```python
from build123d import *

# Parameters (mm, degrees)
F0_R     = 4.35
F0_R_2   = 5
F1_DEPTH = 4.3


with BuildPart() as f1:
    # F0 (on Right) → F1 (new body)
    with BuildSketch(Plane.YZ):
        with BuildLine():
            Line((-22.1, 0), (-5, 0))
            ThreePointArc((-5, 0), (-1.464466, 1.464466), (0, 5))
            Line((0, 5), (0, 29.037729))
            ThreePointArc((0, 29.037729), (-0.662326, 31.524611), (-2.473833, 33.352642))
            Line((-2.473833, 33.352642), (-32.57476, 50.975239))
            ThreePointArc((-32.57476, 50.975239), (-33.70512, 51.245677), (-34.79499, 50.841905))
            Line((-34.79499, 50.841905), (-42.052337, 45.329218))
            Line((-42.052337, 45.329218), (-98.45379, 75.262621))
            ThreePointArc((-98.45379, 75.262621), (-98.549794, 75.301433), (-98.651734, 75.319636))
            Line((-98.651734, 75.319636), (-104.857779, 75.773284))
            ThreePointArc((-104.857779, 75.773284), (-104.881835, 75.769417), (-104.901607, 75.755178))
            ThreePointArc((-104.901607, 75.755178), (-104.997551, 75.587599), (-105.022838, 75.396161))
            Line((-105.022838, 75.396161), (-104.855972, 72.750564))
            ThreePointArc((-104.855972, 72.750564), (-104.882304, 72.556066), (-104.98147, 72.386689))
            ThreePointArc((-104.98147, 72.386689), (-105.0797, 72.27604), (-105.177659, 72.165152))
            ThreePointArc((-105.177659, 72.165152), (-105.519248, 71.996856), (-105.880288, 72.117919))
            Line((-105.880288, 72.117919), (-107.19123, 73.254305))
            ThreePointArc((-107.19123, 73.254305), (-107.768907, 72.57831), (-108.336982, 71.894228))
            ThreePointArc((-108.336982, 71.894228), (-108.432061, 71.710527), (-108.44465, 71.504063))
            Line((-108.44465, 71.504063), (-108.056233, 68.888956))
            ThreePointArc((-108.056233, 68.888956), (-108.06619, 68.692429), (-108.151209, 68.514964))
            ThreePointArc((-108.151209, 68.514964), (-108.239818, 68.396849), (-108.328139, 68.27852))
            ThreePointArc((-108.328139, 68.27852), (-108.65472, 68.082686), (-109.024498, 68.17363))
            Line((-109.024498, 68.17363), (-110.424503, 69.198289))
            ThreePointArc((-110.424503, 69.198289), (-110.941832, 68.480942), (-111.449037, 67.756402))
            ThreePointArc((-111.449037, 67.756402), (-111.530067, 67.558002), (-111.520592, 67.343902))
            Line((-111.520592, 67.343902), (-110.867678, 64.891617))
            ThreePointArc((-110.867678, 64.891617), (-110.856617, 64.687221), (-110.92839, 64.495521))
            ThreePointArc((-110.92839, 64.495521), (-111.004676, 64.374709), (-111.080678, 64.253718))
            ThreePointArc((-111.080678, 64.253718), (-111.390502, 64.032323), (-111.766382, 64.093319))
            Line((-111.766382, 64.093319), (-113.244054, 65.002399))
            ThreePointArc((-113.244054, 65.002399), (-113.70347, 64.243719), (-114.152157, 63.478645))
            ThreePointArc((-114.152157, 63.478645), (-114.216631, 63.278226), (-114.192891, 63.069034))
            Line((-114.192891, 63.069034), (-113.365453, 60.614331))
            ThreePointArc((-113.365453, 60.614331), (-113.340818, 60.415154), (-113.396489, 60.222336))
            ThreePointArc((-113.396489, 60.222336), (-113.463838, 60.093583), (-113.53088, 59.964669))
            ThreePointArc((-113.53088, 59.964669), (-113.821693, 59.718835), (-114.201286, 59.749091))
            Line((-114.201286, 59.749091), (-115.74793, 60.535116))
            ThreePointArc((-115.74793, 60.535116), (-116.14419, 59.74162), (-116.529237, 58.942622))
            ThreePointArc((-116.529237, 58.942622), (-116.577215, 58.737628), (-116.536559, 58.531056))
            Line((-116.536559, 58.531056), (-115.512428, 56.151691))
            ThreePointArc((-115.512428, 56.151691), (-115.471694, 55.955174), (-115.511515, 55.758471))
            ThreePointArc((-115.511515, 55.758471), (-115.568182, 55.624671), (-115.624528, 55.490737))
            ThreePointArc((-115.624528, 55.490737), (-115.894408, 55.222089), (-116.275204, 55.221406))
            Line((-116.275204, 55.221406), (-117.880594, 55.879179))
            Line((-117.880594, 55.879179), (-118.52994, 54.228474))
            ThreePointArc((-118.52994, 54.228474), (-118.561106, 54.020259), (-118.503801, 53.817674))
            Line((-118.503801, 53.817674), (-117.28975, 51.529377))
            ThreePointArc((-117.28975, 51.529377), (-117.233185, 51.336819), (-117.256894, 51.137531))
            ThreePointArc((-117.256894, 51.137531), (-117.302503, 50.99957), (-117.347782, 50.861501))
            ThreePointArc((-117.347782, 50.861501), (-117.594943, 50.571815), (-117.974426, 50.540197))
            Line((-117.974426, 50.540197), (-119.627948, 51.06537))
            ThreePointArc((-119.627948, 51.06537), (-119.890472, 50.218175), (-120.141039, 49.367367))
            ThreePointArc((-120.141039, 49.367367), (-120.155186, 49.157308), (-120.081612, 48.960048))
            Line((-120.081612, 48.960048), (-118.684637, 46.776338))
            ThreePointArc((-118.684637, 46.776338), (-118.61281, 46.590175), (-118.619501, 46.390749))
            Line((-118.619501, 46.390749), (-118.68725, 46.107071))
            ThreePointArc((-118.68725, 46.107071), (-118.910066, 45.798287), (-119.285711, 45.735952))
            Line((-119.285711, 45.735952), (-120.978439, 46.125513))
            Line((-120.978439, 46.125513), (-121.351884, 44.391438))
            ThreePointArc((-121.351884, 44.391438), (-121.348918, 44.180925), (-121.259561, 43.990294))
            Line((-121.259561, 43.990294), (-119.690523, 41.928256))
            ThreePointArc((-119.690523, 41.928256), (-119.606388, 41.758287), (-119.591605, 41.569211))
            ThreePointArc((-119.591605, 41.569211), (-119.592977, 41.558197), (-119.594592, 41.547217))
            Line((-119.594592, 41.547217), (-119.640055, 41.26036))
            ThreePointArc((-119.640055, 41.26036), (-119.83704, 40.934471), (-120.206393, 40.841815))
            Line((-120.206393, 40.841815), (-121.923138, 41.092269))
            ThreePointArc((-121.923138, 41.092269), (-122.041201, 40.24253), (-122.147679, 39.391262))
            ThreePointArc((-122.147679, 39.391262), (-122.110207, 39.260888), (-122.03907, 39.145384))
            Line((-122.03907, 39.145384), (-120.283735, 37.010276))
            ThreePointArc((-120.283735, 37.010276), (-120.193147, 36.843224), (-120.171435, 36.654436))
            ThreePointArc((-120.171435, 36.654436), (-120.182866, 36.503198), (-120.19392, 36.351932))
            ThreePointArc((-120.19392, 36.351932), (-120.363778, 36.011117), (-120.724382, 35.888759))
            Line((-120.724382, 35.888759), (-122.472888, 36))
            Line((-122.472888, 36), (-131.6, 36))
            Line((-131.6, 36), (-131.6, 5))
            ThreePointArc((-131.6, 5), (-130.135534, 1.464466), (-126.6, 0))
            Line((-126.6, 0), (-109.5, 0))
            ThreePointArc((-109.5, 0), (-105.964466, 1.464466), (-104.5, 5))
            Line((-104.5, 5), (-104.5, 16.84052))
            ThreePointArc((-104.5, 16.84052), (-104.025137, 18.967287), (-102.690745, 20.690085))
            Line((-102.690745, 20.690085), (-91.09576, 30.300687))
            ThreePointArc((-91.09576, 30.300687), (-89.600918, 31.154729), (-87.905015, 31.451123))
            Line((-87.905015, 31.451123), (-83.976422, 31.451123))
            ThreePointArc((-83.976422, 31.451123), (-80.857839, 30.359375), (-79.101138, 27.560898))
            ThreePointArc((-79.101138, 27.560898), (-59.369338, 12.00133), (-40.001664, 28.011865))
            ThreePointArc((-40.001664, 28.011865), (-38.26553, 30.886857), (-35.10208, 32.014832))
            Line((-35.10208, 32.014832), (-32.1, 32.014832))
            ThreePointArc((-32.1, 32.014832), (-28.564466, 30.550365), (-27.1, 27.014832))
            Line((-27.1, 27.014832), (-27.1, 5))
            ThreePointArc((-27.1, 5), (-25.635534, 1.464466), (-22.1, 0))
        make_face()
        with Locations((-118.05, 9.35)):
            Circle(F0_R, mode=Mode.SUBTRACT)
        with Locations((-13.55, 9.35)):
            Circle(F0_R, mode=Mode.SUBTRACT)
        with Locations((-59.6, 32)):
            Circle(F0_R_2, mode=Mode.SUBTRACT)
    extrude(amount=F1_DEPTH)


solid = f1.part
```
Geometry check sheet. Reference: the model listing, model coordinates, mm. A direction names the side the tool comes from. Coordinates: 2 decimals unless noted, no trailing zeros. Write each loop counter-clockwise with the first axis right and the second up, starting at its lowest first coordinate (ties: lowest second). Pieces come first, ordered by that corner, then holes. Notation, with made-up numbers: M 54,0 L 93,0 A23 ccw 93,11 Z; hole C 63,60 d3. An arc over 180 degrees is marked long. One line per item, written item: value. Start each with the question number.
(1) Sectioned sample at A-A, the plane z = 9.35. Enter the section's corners in (x, y), and give its area (3 significant figures).
(2) Depth check by flat-ended pin: pin 1 (2 mm diameter, centred on x = 2, y = -127, fed in from +Z); pin 2 (1.5 mm diameter, centred on x = 2.5, z = 50.5, fed in from -Y); pin 3 (2 mm diameter, centred on x = 2.5, y = -86.5, fed in from -Z). Enter the tip coordinate at first touch or a pass-through.
(3) Sectioned sample at D-D, the plane y = -13.55. Enter the section's corners in (x, z), and give its area (3 significant figures).
(4) Sectioned sample at B-B, the plane y = -59.6. Enter the section's corners in (x, z), and give its area (3 significant figures).
(5) Sectioned sample at C-C, the plane x = 3.4. State how many separate pieces and enclosed holes the cut face has, and give its area (3 significant figures).
(6) Tool access check on faces 1 (the face through (2.12, -116.032, 57.358)), 2 (the face through (2.12, -104.04, 18.94)), 3 (the face through (2.12, -69.858, 60.086)). Record the directions out of +Z, -Z, +X, -X, +Y, -Y that give a thin tool (end or side, any length) a straight path to the whole face; none if there is none.
(7) Scan lines: line 1 along Y through (x, z) = (1.55, 22); line 2 along Z through (x, y) = (2.1, -123.5); line 3 along Y through (x, z) = (0.3, 3). Record each from-to range of solid material in increasing order. Write a range as [from, to].
(8) Release check for a two-part mould opening along Z. For faces 4 (the face through (2.1, -113.8, 61.9)), 5 (the face through (2, -104.5, 11)), 6 (the face through (2.1, -59.7, 12)) record: released by +Z, released by -Z, zero draft, split by the parting line, or undercut.
Filled sheet:
1. outline: M 0,-131.6 L 4.3,-131.6 L 4.3,-122.4 L 0,-122.4 Z; M 0,-113.7 L 4.3,-113.7 L 4.3,-104.5 L 0,-104.5 Z; M 0,-27.1 L 4.3,-27.1 L 4.3,-17.9 L 0,-17.9 Z; M 0,-9.2 L 4.3,-9.2 L 4.3,0 L 0,0 Z
1. area: 158 mm²
2. pin 1: z = 36
2. pin 2: y = -120.03
2. pin 3: z = 31.45
3. outline: M 0,0 L 4.3,0 L 4.3,5 L 0,5 Z; M 0,13.7 L 4.3,13.7 L 4.3,39.84 L 0,39.84 Z
3. area: 134 mm²
4. outline: M 0,12 L 4.3,12 L 4.3,27 L 0,27 Z; M 0,37 L 4.3,37 L 4.3,54.64 L 0,54.64 Z
4. area: 140 mm²
5. separate pieces: 1
5. enclosed holes: 3
5. area: 5,130 mm²
6. face 1: +X, -X, -Y
6. face 2: -Z, +X, -X
6. face 3: +Z, +X, -X
7. line 1: [-131.6, -101.11], [-76.92, -42.28], [-27.1, 0]
7. line 2: [0, 36]
7. line 3: [-131.18, -104.92], [-26.68, -0.42]
8. face 4: undercut
8. face 5: zero draft
8. face 6: released by -Z
